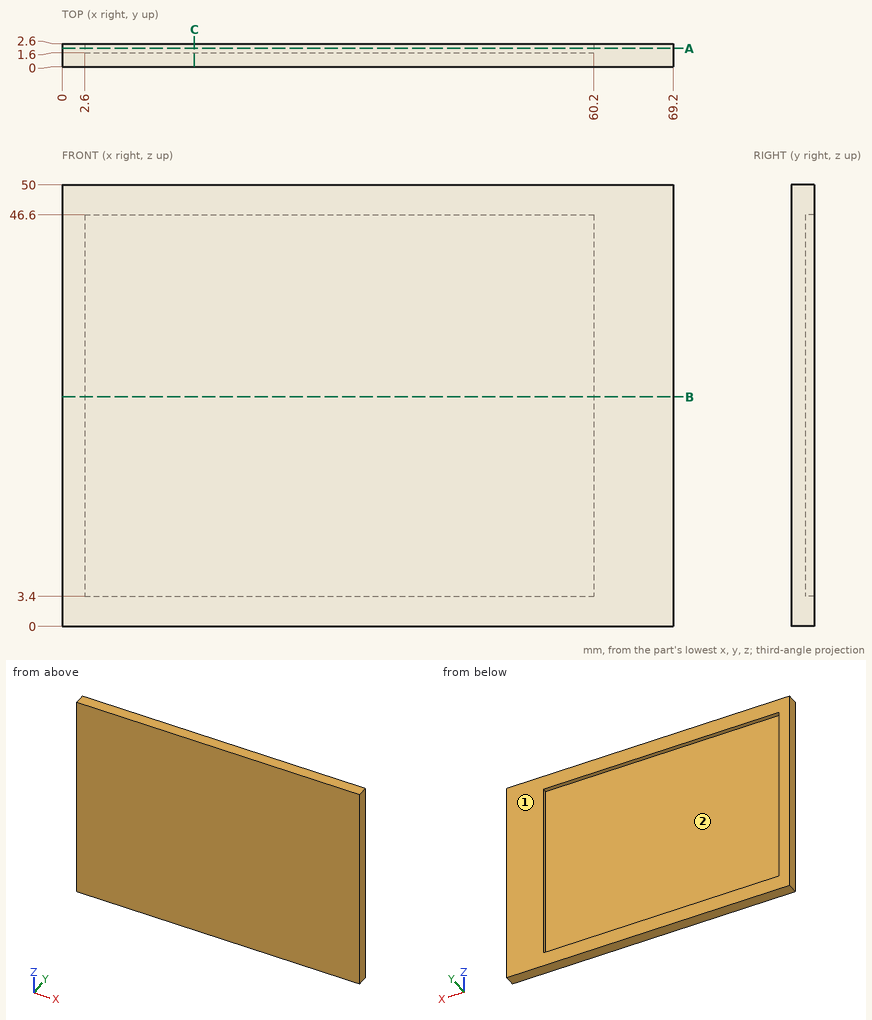
Check sheet for the drawn part. Datum: minimum x, y, z corner. Units: mm. Give positions to 0.01 mm unless a question says otherwise; leave off trailing zeros. Order: outer loops, then holes, each group sorted by start corner. A loop starts at its lowest first (then second) coordinate and runs counter-clockwise, first axis right, second up. Notation, with made-up numbers: (30.5, 85.25) -> (76.5, 85.25) arc R30 ccw to (76.5, 123.25) -> close; hole circle Ø8 at (2, -15.75). An arc over 180 degrees is marked (long way). Use a Markdown table: item, result.
1) Material ranges on probe 1 along X at (y, z) = (2, 24); probe 2 along Z at (x, y) = (30.5, 2.25); probe 3 along Y at (x, z) = (51, 4), recorded low to high.
Results:
| item | result |
|---|---|
| probe 1 | 0 to 2.6, 60.2 to 69.2 |
| probe 2 | 0 to 3.4, 46.6 to 50 |
| probe 3 | 0 to 1.6 |
2) Depth check by flat-ended pin: pin 1 Ø3 at (x, z) = (8.5, 21.5) entering from +Y. Enter the tip coordinate at first touch or a pass-through.
Results:
| item | result |
|---|---|
| pin 1 | y = 1.6 |
3) Mould release check, pull along Z, two halves, no side actions. Record for the marked faces 1 and 2: pulls with the +Z half, pulls with the -Z half, needs draft (parallel to the pull), parting line crosses it, or undercut.
Results:
| item | result |
|---|---|
| face 1 | needs draft |
| face 2 | undercut |
4) Section check A-A, the plane y = 2.1. Record the boundary of the cut face in (x, z).
Results:
| item | result |
|---|---|
| outline | (0, 0) -> (69.2, 0) -> (69.2, 50) -> (0, 50) -> close; hole (2.6, 3.4) -> (60.2, 3.4) -> (60.2, 46.6) -> (2.6, 46.6) -> close |
5) Section check C-C, the plane x = 15. Record the boundary of the cut face in (y, z).
Results:
| item | result |
|---|---|
| outline | (0, 0) -> (2.6, 0) -> (2.6, 3.4) -> (1.6, 3.4) -> (1.6, 46.6) -> (2.6, 46.6) -> (2.6, 50) -> (0, 50) -> close |
6) Section check B-B, the plane z = 26. Record the boundary of the cut face in (x, y), then the cut area to 3 significant figures.
Results:
| item | result |
|---|---|
| outline | (0, 0) -> (69.2, 0) -> (69.2, 2.6) -> (60.2, 2.6) -> (60.2, 1.6) -> (2.6, 1.6) -> (2.6, 2.6) -> (0, 2.6) -> close |
| area | 122 mm² |
